Source: CAD feature listing. Evaluate the final solid. Frame: model axes, mm. Round coordinates to 2 decimals unless told otherwise and drop trailing zeros. Order: outer loops, then holes, each group sorted by start corner. A loop starts at its lowest first (then second) coordinate and runs counter-clockwise, first axis right, second up. Notation, with made-up numbers: (1, -19) -> (12, -19) arc R24 cw to (12, 12) -> close; hole circle Ø2 at (25.25, 57.25). An arc over 180 degrees is marked (long way). Write item = value, one per line. Start each with the question number.
(1) Cut plane C-C on z = -31. Return the cut outline in (x, y), then the cut area to 3 significant figures.
(2) Ray query, line 1 (Z direction, x = 28, y = 0.5); line 2 (Z direction, x = 38.5, y = 0.8); line 3 (X direction, y = 0.15, z = -33). Return the intervals inside material, ascending.
(3) Cut plane B-B on x = 38.5. Return the cut outline in (y, z), then the cut area to 3 significant figures.
(4) Cut plane A-A on y = 0.2. Return the cut outline in (x, z) (3 decimals), then the cut area to 3 significant figures.
from build123d import *

# Parameters (mm, degrees)
BOSS_EXTRUDE1_DEPTH = 1.00076


with BuildPart() as part:
    # Sketch3 → Boss-Extrude1 (new body)
    with BuildSketch(Plane(origin=(0, 0, 0), x_dir=(1, 0, 0), z_dir=(0, 1, 0))):
        with BuildLine():
            Line((0, 63.5), (0, 0))
            Line((0, 0), (24.257, 0))
            Line((24.257, 0), (24.257, 10.953386454))
            ThreePointArc((24.257, 10.953386454), (7.334843244, 31.75), (24.257, 52.546613546))
            Line((24.257, 52.546613546), (24.257, 63.5))
            Line((24.257, 63.5), (0, 63.5))
        make_face()
        with BuildLine():
            Line((32.893, 10.953386454), (32.893, 0))
            Line((32.893, 0), (52.07, 0))
            Line((52.07, 0), (52.07, 63.5))
            Line((52.07, 63.5), (32.893, 63.5))
            Line((32.893, 63.5), (32.893, 52.546613546))
            ThreePointArc((32.893, 52.546613546), (45.050121485, 45.155768574), (49.815156756, 31.75))
            ThreePointArc((49.815156756, 31.75), (45.050121485, 18.344231426), (32.893, 10.953386454))
        make_face()
        with BuildLine():
            Line((28.575, 10.509843244), (28.575, 0))
            Line((28.575, 0), (32.893, 0))
            Line((32.893, 0), (32.893, 10.953386454))
            ThreePointArc((32.893, 10.953386454), (30.745360257, 10.621020011), (28.575, 10.509843244))
        make_face()
        with BuildLine():
            Line((24.257, 10.953386454), (24.257, 0))
            Line((24.257, 0), (28.575, 0))
            Line((28.575, 0), (28.575, 10.509843244))
            ThreePointArc((28.575, 10.509843244), (26.404639743, 10.621020011), (24.257, 10.953386454))
        make_face()
        with BuildLine():
            Line((32.893, 63.5), (28.575, 63.5))
            Line((28.575, 63.5), (28.575, 52.990156756))
            ThreePointArc((28.575, 52.990156756), (30.745360257, 52.878979989), (32.893, 52.546613546))
            Line((32.893, 52.546613546), (32.893, 63.5))
        make_face()
        with BuildLine():
            Line((28.575, 63.5), (24.257, 63.5))
            Line((24.257, 63.5), (24.257, 52.546613546))
            ThreePointArc((24.257, 52.546613546), (26.404639743, 52.878979989), (28.575, 52.990156756))
            Line((28.575, 52.990156756), (28.575, 63.5))
        make_face()
    extrude(amount=BOSS_EXTRUDE1_DEPTH)


solid = part.part
Evaluation:
q1.outline = (0, 0) -> (7.35, 0) -> (7.35, 1) -> (0, 1) -> close; (49.8, 0) -> (52.07, 0) -> (52.07, 1) -> (49.8, 1) -> close
q1.area = 9.62 mm^2
q2.line_1 = -63.5 to -52.98, -10.52 to 0
q2.line_2 = -63.5 to -50.53, -12.97 to 0
q2.line_3 = 0 to 7.37, 49.78 to 52.07
q3.outline = (0, -63.5) -> (1, -63.5) -> (1, -50.53) -> (0, -50.53) -> close; (0, -12.97) -> (1, -12.97) -> (1, 0) -> (0, 0) -> close
q3.area = 26.0 mm^2
q4.outline = (0, -63.5) -> (52.07, -63.5) -> (52.07, 0) -> (0, 0) -> close; hole circle Ø42.48 at (28.575, -31.75)
q4.area = 1,890 mm^2
